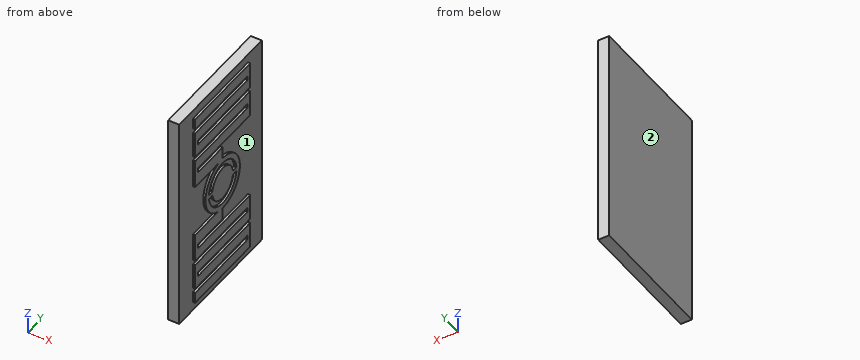
Autodesk Inventor part; units mm, degrees
ref_plane "YZ Plane" through (0, 0, 0) normal (1, 0, 0) x (0, 1, 0)
ref_plane "XZ Plane" through (0, 0, 0) normal (0, 1, 0) x (-1, 0, 0)
ref_plane "XY Plane" through (0, 0, 0) normal (0, 0, 1) x (1, 0, 0)
sketch "Sketch1" plane through (0, 0, 0) normal (1, 0, 0) x (0, 1, 0)
  line L0 (-3, 5) -> (3, 5)
  line L1 (3, 5) -> (3, -5)
  line L2 (3, -5) -> (-3, -5)
  line L3 (-3, -5) -> (-3, 5)
  point P0 (0, 0)
  dimension "d0" = 6
  dimension "d1" = 10
  dimension "d2" = 3
  dimension "d3" = 5
extrude "Extrusion1" add sketch "Sketch1" along normal blind 0.5
sketch "Sketch2" plane through (0.5, 0, 0) normal (1, 0, 0) x (0, 0, -1)
  circle A0 centre (0, 0) radius 0.75
  circle A1 centre (0, 0) radius 1
  circle A2 centre (0, 0) radius 1.25
  line L0 (-2.5, -2) -> (-2, -2)
  line L1 (-2, -2) -> (-2, 2)
  line L2 (-2, 2) -> (-2.5, 2)
  line L3 (-2.5, 2) -> (-2.5, -2)
  line L4 (-5, -3) -> (5, -3)
  line L5 (-3.2, -2) -> (-2.7, -2)
  line L6 (-2.7, -2) -> (-2.7, 2)
  line L7 (-2.7, 2) -> (-3.2, 2)
  line L8 (-3.2, 2) -> (-3.2, -2)
  line L9 (-3.9, -2) -> (-3.4, -2)
  line L10 (-3.4, -2) -> (-3.4, 2)
  line L11 (-3.4, 2) -> (-3.9, 2)
  line L12 (-3.9, 2) -> (-3.9, -2)
  line L13 (-4.6, -2) -> (-4.1, -2)
  line L14 (-4.1, -2) -> (-4.1, 2)
  line L15 (-4.1, 2) -> (-4.6, 2)
  line L16 (-4.6, 2) -> (-4.6, -2)
  line L17 (-0.1, -1.1173) -> (0.1, -1.1173)
  line L18 (0.1, -1.1173) -> (0.1, 1.1584)
  line L19 (0.1, 1.1584) -> (-0.1, 1.1584)
  line L20 (-0.1, 1.1584) -> (-0.1, -1.1173)
  line L21 (-1.8, -2) -> (-1.2, -2)
  line L22 (-1.2, -2) -> (-1.2, 0)
  line L23 (-1.2, 0) -> (-1.8, 0)
  line L24 (-1.8, 0) -> (-1.8, -2)
  line L25 (-1.8, -2) -> (-2, -2)
  line L26 (-2, -2) -> (-2, -1.8)
  line L27 (-2, -1.8) -> (-1.8, -1.8)
  line L28 (-1.8, -1.8) -> (-1.8, -2)
  line L29 (-2.5, 2) -> (-2.7, 2)
  line L30 (-2.7, 2) -> (-2.7, 1.8)
  line L31 (-2.7, 1.8) -> (-2.5, 1.8)
  line L32 (-2.5, 1.8) -> (-2.5, 2)
  line L33 (-3.2, -2) -> (-3.4, -2)
  line L34 (-3.4, -2) -> (-3.4, -1.8)
  line L35 (-3.4, -1.8) -> (-3.2, -1.8)
  line L36 (-3.2, -1.8) -> (-3.2, -2)
  line L37 (-3.9, 2) -> (-4.1, 2)
  line L38 (-4.1, 2) -> (-4.1, 1.8)
  line L39 (-4.1, 1.8) -> (-3.9, 1.8)
  line L40 (-3.9, 1.8) -> (-3.9, 2)
  line L41 (0, -3) -> (0, -2)
  circle A3 centre (0, 0) radius 0.75
  circle A4 centre (0, 0) radius 1
  circle A5 centre (0, 0) radius 1.25
  line L42 (2.5, -2) -> (2, -2)
  line L43 (2, -2) -> (2, 2)
  line L44 (2, 2) -> (2.5, 2)
  line L45 (2.5, 2) -> (2.5, -2)
  line L46 (3.2, -2) -> (2.7, -2)
  line L47 (2.7, -2) -> (2.7, 2)
  line L48 (2.7, 2) -> (3.2, 2)
  line L49 (3.2, 2) -> (3.2, -2)
  line L50 (3.9, -2) -> (3.4, -2)
  line L51 (3.4, -2) -> (3.4, 2)
  line L52 (3.4, 2) -> (3.9, 2)
  line L53 (3.9, 2) -> (3.9, -2)
  line L54 (4.6, -2) -> (4.1, -2)
  line L55 (4.1, -2) -> (4.1, 2)
  line L56 (4.1, 2) -> (4.6, 2)
  line L57 (4.6, 2) -> (4.6, -2)
  line L58 (0.1, -1.1173) -> (-0.1, -1.1173)
  line L59 (-0.1, -1.1173) -> (-0.1, 1.1584)
  line L60 (-0.1, 1.1584) -> (0.1, 1.1584)
  line L61 (0.1, 1.1584) -> (0.1, -1.1173)
  line L62 (1.8, -2) -> (1.2, -2)
  line L63 (1.2, -2) -> (1.2, 0)
  line L64 (1.2, 0) -> (1.8, 0)
  line L65 (1.8, 0) -> (1.8, -2)
  line L66 (1.8, -2) -> (2, -2)
  line L67 (2, -2) -> (2, -1.8)
  line L68 (2, -1.8) -> (1.8, -1.8)
  line L69 (1.8, -1.8) -> (1.8, -2)
  line L70 (2.5, 2) -> (2.7, 2)
  line L71 (2.7, 2) -> (2.7, 1.8)
  line L72 (2.7, 1.8) -> (2.5, 1.8)
  line L73 (2.5, 1.8) -> (2.5, 2)
  line L74 (3.2, -2) -> (3.4, -2)
  line L75 (3.4, -2) -> (3.4, -1.8)
  line L76 (3.4, -1.8) -> (3.2, -1.8)
  line L77 (3.2, -1.8) -> (3.2, -2)
  line L78 (3.9, 2) -> (4.1, 2)
  line L79 (4.1, 2) -> (4.1, 1.8)
  line L80 (4.1, 1.8) -> (3.9, 1.8)
  line L81 (3.9, 1.8) -> (3.9, 2)
  dimension "d6" = 1.5
  dimension "d7" = 2
  dimension "d8" = 2.5
  dimension "d9" = 0.5
  dimension "d10" = 4
  dimension "d11" = 1
  dimension "d14" = 0.7
  dimension "d19" = 0.2
  dimension "d20" = 0.1
  dimension "d21" = 2
  dimension "d22" = 0.6
  dimension "d23" = 2
  dimension "d24" = 0.2
  dimension "d25" = 0.2
  dimension "d26" = 0.2
  dimension "d27" = 0.2
  dimension "d28" = 0.2
extrude "Extrusion2" add sketch "Sketch2" along normal blind 0.1 contours A0 L18 | L18 A0 L20 | A0 L20 A1 L18 | L18 A1 L20 A0 | L20 A0 | A1 L20 L19 L18 | L18 L17 L20 A1 | L64 L63 A2 L22 L23 | L64 L65 L62 L63 A2 | A2 L63 L64 | L23 L22 A2 | A2 L22 L21 L24 L23 | L68 L43 L66 L65 | L24 L25 L1 L27 | L43 L44 L45 L42 | L1 L0 L3 L2 | L70 L47 L72 L45 | L3 L31 L6 L29 | L48 L49 L46 L47 | L6 L5 L8 L7 | L76 L51 L74 L49 | L8 L33 L10 L35 | L51 L52 L53 L50 | L10 L9 L12 L11 | L78 L55 L80 L53 | L12 L39 L14 L37 | L56 L57 L54 L55 | L14 L13 L16 L15
properties part number "MEMS"
The listing builds one solid part. Answer for the finished solid, in the listing's coordinates (mm). Face numbers are marked on the shaded views. Coordinates: 2 decimals unless noted, no trailing zeros. Order: outer loops, then holes, each group sorted by start corner. A loop starts at its lowest first (then second) coordinate and runs counter-clockwise, first axis right, second up.
Q1. A cutting plane is placed at C-C, the plane z = 3.75. Write down the section's boundary in (x, y).
Q2. A cutting plane is placed at A-A, the plane z = -4. Write down the section's boundary in (x, y), and give its area (3 significant figures).
Q3. For a pull along Z with two mould halves and no side action, classify the marked faces 1 and 2 as pulls with the +Z half, pulls with the -Z half, needs draft (parallel to the pull), parting line crosses it, or undercut.
Q4. A cutting plane is placed at D-D, the plane z = 0.25. Write down the section's boundary in (x, y).
Q5. Consider line 1 (X direction, y = 0.7, z = 4); line 2 (Y direction, x = 0.55, z = -1.5). Determine where each line is inside the solid, lowest interval first.
Q6. A cutting plane is placed at B-B, the plane y = -2.3. Write down the section's boundary in (x, z).
Answers follow:
1. outline: (0, -3) - (0.5, -3) - (0.5, -2) - (0.6, -2) - (0.6, 2) - (0.5, 2) - (0.5, 3) - (0, 3) - close
2. outline: (0, -3) - (0.5, -3) - (0.5, 1.8) - (0.6, 1.8) - (0.6, 2) - (0.5, 2) - (0.5, 3) - (0, 3) - close
2. area: 3.02 mm2
3. face 1: undercut
3. face 2: needs draft
4. outline: (0, -3) - (0.5, -3) - (0.5, -1.22) - (0.6, -1.22) - (0.6, -0.97) - (0.5, -0.97) - (0.5, -0.71) - (0.6, -0.71) - (0.6, 0.71) - (0.5, 0.71) - (0.5, 0.97) - (0.6, 0.97) - (0.6, 1.22) - (0.5, 1.22) - (0.5, 3) - (0, 3) - close
5. line 1: x = 0 to 0.5
5. line 2: y = -2 to 0
6. outline: (0, -5) - (0.5, -5) - (0.5, 5) - (0, 5) - close
